```python
from build123d import *

# Parameters (mm, degrees)
F0_W     = 118.0035807192
F0_H     = 75.6891593337
F1_DEPTH = 50.8
F2_W     = 99.5282679796
F2_H     = 34.2687154189
F3_DEPTH = 75.6901593337
F4_W     = 70.3253671527
F4_H     = 30.096870847
F4_H_2   = 7.7477134764
F5_DEPTH = 50.801
F6_R     = 10.5691557052
F7_DEPTH = 118.0045807192


with BuildPart() as f1:
    # F0 (on Front) → F1 (new body)
    with BuildSketch(Plane.XZ):
        with Locations((4.1718464345, 3.1288824975)):
            Rectangle(F0_W, F0_H)
    extrude(amount=F1_DEPTH)

    # F2 (on face) → F3 (cut, through all)
    with BuildSketch(Plane(origin=(0, 0, -34.7156971693), x_dir=(1, 0, 0), z_dir=(0, 0, -1))):
        with Locations((3.277875483, 24.4350838475)):
            Rectangle(F2_W, F2_H)
    extrude(amount=-F3_DEPTH, mode=Mode.SUBTRACT)

    # F4 (on face) → F5 (cut, through all)
    with BuildSketch(Plane.XZ.offset(50.8)):
        with Locations((4.4698342681, 25.9250267409)):
            Rectangle(F4_W, F4_H)
        with Locations((4.4698342681, 44.8473189026)):
            Rectangle(F4_W, F4_H_2)
    extrude(amount=-F5_DEPTH, mode=Mode.SUBTRACT)

    # F6 (on face) → F7 (cut, through all)
    with BuildSketch(Plane.YZ.offset(63.1736367941)):
        with Locations((-25.6270393729, 5.8107818477)):
            Circle(F6_R)
    extrude(amount=-F7_DEPTH, mode=Mode.SUBTRACT)


solid = f1.part
```
Verification items for the finished model (mm, model axes). A direction names the side the tool comes from. Coordinates: 2 decimals unless noted, no trailing zeros. Order: outer loops, then holes, each group sorted by start corner. A loop starts at its lowest first (then second) coordinate and runs counter-clockwise, first axis right, second up. Notation, with made-up numbers: (9.5, -35.75) - (24.5, -35.75) arc R26 cw to (24.5, 3.25) - close; hole circle Ø11 at (69.25, 51). An arc over 180 degrees is marked (long way). Return JSON: item names as keys, results as strings.
(1) Section check D-D, the plane z = -26. Record the cut outline in (x, y).
Filled sheet:
{"outline": "(-54.83, -50.8) - (63.17, -50.8) - (63.17, 0) - (-54.83, 0) - close; hole (-46.49, -41.57) - (53.04, -41.57) - (53.04, -7.3) - (-46.49, -7.3) - close"}
(2) Thickness scan on line 1 along Y through (x, z) = (51, -28); line 2 along X through (y, z) = (-30.5, -11); line 3 along X through (y, z) = (-43, 32). Record the ranges inside material, lowest first.
Filled sheet:
{"line 1": "y = -50.8 to -41.57, -7.3 to 0", "line 2": "x = -54.83 to -46.49, 53.04 to 63.17", "line 3": "x = -54.83 to -30.69, 39.63 to 63.17"}
(3) Section check C-C, the plane y = -10. Record the cut outline in (x, z).
Filled sheet:
{"outline": "(-54.83, -34.72) - (-46.49, -34.72) - (-46.49, 40.97) - (-54.83, 40.97) - close; (53.04, -34.72) - (63.17, -34.72) - (63.17, 40.97) - (53.04, 40.97) - close"}
(4) Mould release check, pull along X, two halves, no side actions. Record for faces 1 (the flat face through (-54.83, -25, -6)), 2 (the flat face through (53.042, -24, -6)), 3 (the flat face through (3, -7.301, -6)), 4 (the flat face through (3, 0, -5)): pulls with the +X half, pulls with the -X half, needs draft (parallel to the pull), parting line crosses it, or undercut.
Filled sheet:
{"face 1": "pulls with the -X half", "face 2": "undercut", "face 3": "undercut", "face 4": "needs draft"}
(5) Section check B-B, the plane x = -43.5. Record the cut outline in (y, z).
Filled sheet:
{"outline": "(-50.8, -34.72) - (-41.57, -34.72) - (-41.57, 40.97) - (-50.8, 40.97) - close; (-7.3, -34.72) - (0, -34.72) - (0, 40.97) - (-7.3, 40.97) - close"}
(6) Section check A-A, the plane z = 32.5. Record the cut outline in (x, y), and give its area (3 significant figures).
Filled sheet:
{"outline": "(-54.83, -50.8) - (-30.69, -50.8) - (-30.69, -41.57) - (-46.49, -41.57) - (-46.49, -7.3) - (-30.69, -7.3) - (-30.69, 0) - (-54.83, 0) - close; (39.63, -50.8) - (63.17, -50.8) - (63.17, 0) - (39.63, 0) - (39.63, -7.3) - (53.04, -7.3) - (53.04, -41.57) - (39.63, -41.57) - close", "area": "1,420 mm^2"}
(7) Access from +Z, -Z, +X, -X, +Y, -Y to the whole of each face (thin tool, end or side, straight path). Record for faces 5 (the cylindrical face through (58.179, -15.546, 8.985)), 6 (the flat face through (39.633, -4, 26)), 7 (the flat face through (3, -41.569, -6)).
Filled sheet:
{"face 5": "+X, -X", "face 6": "+Z, +Y, -Y", "face 7": "+Z, -Z"}
(8) Go/stop test with flat-tipped pins: pin 1 (17 mm diameter, centred on y = -25.63, z = 5.81, fed in from +X); pin 2 (2 mm diameter, centred on x = 18, y = -5, fed in from +Z). Record where each tip stops, or that it passes through.
Filled sheet:
{"pin 1": "passes through", "pin 2": "stops at z = 10.88"}
